Geometry check sheet. Reference: the model listing, model coordinates, mm. Face numbers are marked on the shaded views. A direction names the side the tool comes from. Coordinates: 2 decimals unless noted, no trailing zeros. Loops run counter-clockwise (first coordinate to the right, second up) from the corner with the lowest first, then second, coordinate; pieces in that order, holes last. Notation, with made-up numbers: (53, -11.75) - (77, -11.75) arc R20 ccw to (77, 22.25) - close; hole circle Ø2 at (-23.75, 52.25). An arc over 180 degrees is marked (long way). One line per item, written item: value.
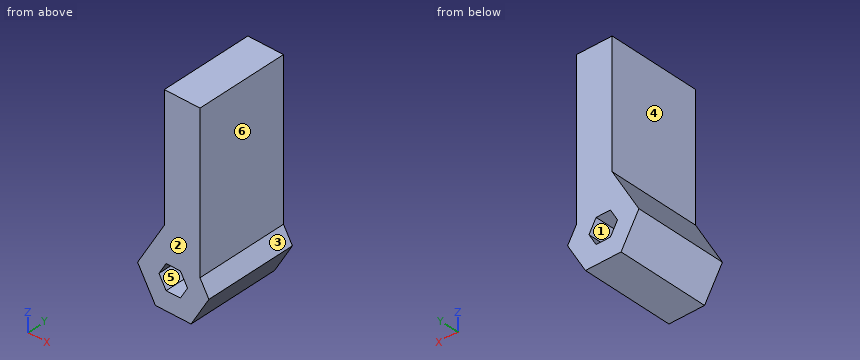
from build123d import *

# Parameters (mm, degrees)
BOSS_EXTRUDE1_DEPTH = 15


with BuildPart() as part:
    # Sketch1 → Boss-Extrude1 (new body)
    with BuildSketch(Plane(origin=(0, 0, 0), x_dir=(1, 0, 0), z_dir=(0, 1, 0))):
        Polygon((-1.443375673, -7.5), (-1.443375673, -27.5), (4.330127019, -27.5), (4.330127019, -2.5), (5.773502692, 0), (2.886751346, 5), (-2.886751346, 5), (-5.773502692, 0), align=None)
        Polygon((2.309401077, 0), (1.154700538, 2), (-1.154700538, 2), (-2.309401077, 0), (-1.154700538, -2), (1.154700538, -2), align=None, mode=Mode.SUBTRACT)
    extrude(amount=BOSS_EXTRUDE1_DEPTH)


solid = part.part
(1) Cross-section at B-B on y = 5.25. Record the cut outline in (x, z), and give its area (3 significant figures).
Reply:
outline: (-5.77, 0) - (-2.89, -5) - (2.89, -5) - (5.77, 0) - (4.33, 2.5) - (4.33, 27.5) - (-1.44, 27.5) - (-1.44, 7.5) - close; hole (-2.31, 0) - (-1.15, -2) - (1.15, -2) - (2.31, 0) - (1.15, 2) - (-1.15, 2) - close
area: 206 mm2
(2) Release check for a two-part mould opening along X. For the marked faces 1, 2 and 3 record: pulls with the +X half, pulls with the -X half, needs draft (parallel to the pull), parting line crosses it, or undercut.
Reply:
face 1: undercut
face 2: needs draft
face 3: pulls with the +X half
(3) Cross-section at D-D on x = -3.75. Record the cut outline in (y, z).
Reply:
outline: (0, -3.5) - (15, -3.5) - (15, 3.5) - (0, 3.5) - close
(4) Cross-section at C-C on z = 5. Record the cut outline in (x, y), and give its area (3 significant figures).
Reply:
outline: (-2.89, 0) - (4.33, 0) - (4.33, 15) - (-2.89, 15) - close
area: 108 mm2
(5) Material ranges on probe 1 along Z at (x, y) = (-0.5, 3.25); probe 2 along X at (y, z) = (1.75, 18); probe 3 along X at (y, z) = (1.5, -1), recorded low to high. Write a range as from..to.
Reply:
probe 1: -5..-2, 2..27.5
probe 2: -1.44..4.33
probe 3: -5.2..-1.73, 1.73..5.2
(6) Go/stop test with flat-tipped pins: pin 1 Ø3 at (y, z) = (10, 18) entering from -X; pin 2 Ø1 at (y, z) = (2.5, 6) entering from -X. Record where each tip stops, or that it passes through.
Reply:
pin 1: x = -1.44
pin 2: x = -2.6
(7) Access from +Z, -Z, +X, -X, +Y, -Y to the whole of each face (thin tool, end or side, straight path). Record for the marked faces 4, 5 and 6.
Reply:
face 4: +Z, -X, +Y, -Y
face 5: +Y, -Y
face 6: +Z, +X, +Y, -Y
(8) Cross-section at A-A on x = 0.5. Record the cut outline in (y, z).
Reply:
outline: (0, -5) - (15, -5) - (15, -2) - (0, -2) - close; (0, 2) - (15, 2) - (15, 27.5) - (0, 27.5) - close
